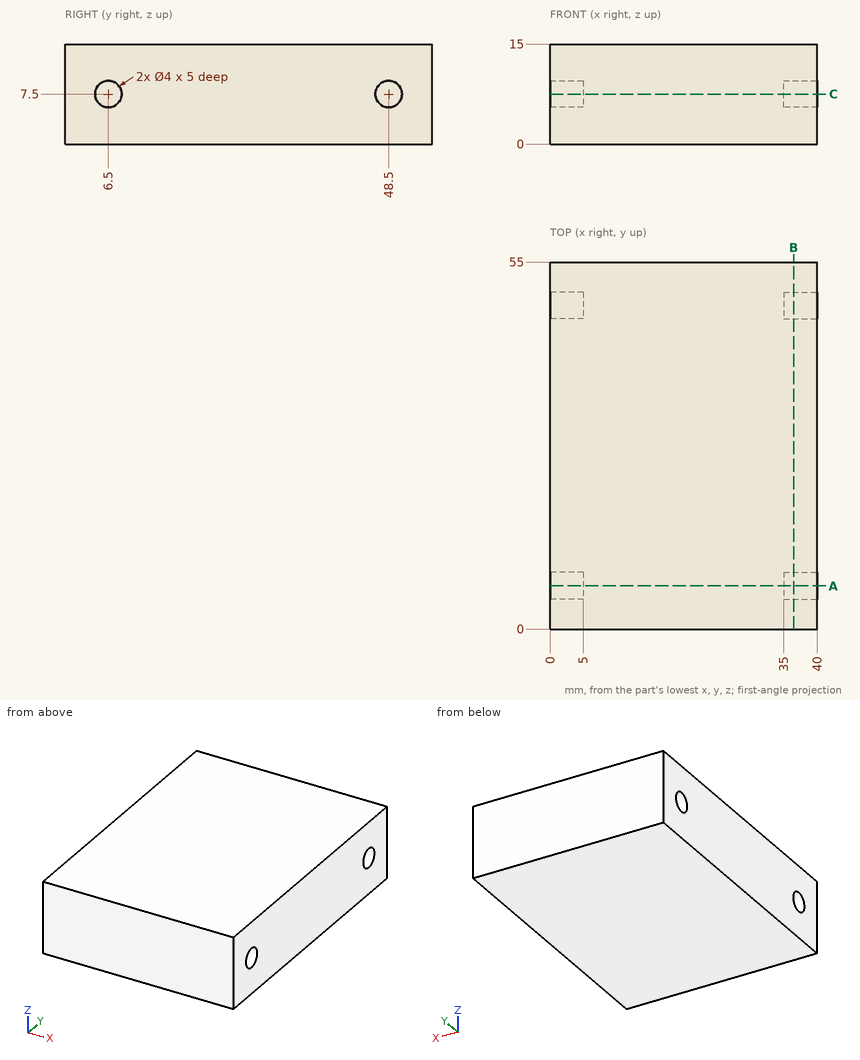
Could you check a few things on this drawing? It's one solid part, dimensions in mm from its lowest x, y, z. Coordinates: 2 decimals unless noted, no trailing zeros. Write each loop counter-clockwise with the first axis right and the second up, starting at its lowest first coordinate (ties: lowest second). Pieces come first, ordered by that corner, then holes. Notation, with made-up numbers: (65.5, -24.75) - (89.5, -24.75) arc R16 cw to (89.5, -19.75) - close; hole circle Ø4 at (11.5, 70.25). An arc over 180 degrees is marked (long way). Put each result on its own line as item: value. Start each with the question number.
Q1. I'm going to push flat-ended pins straight in: P1, Ø2.5, axis at y = 6.5, z = 7.5, coming from the +X side; P2, Ø1.2, axis at y = 49, z = 7, coming from the -X side. Where does each tip first touch, or does it pass through?
Q2. I want a section at C-C on z = 7.5. Write out the boundary of the cut face in (x, y).
Q3. Please list where these lines run through material, in increasing order: L1, parallel to Y at x = 37.45, z = 7.5; L2, parallel to Z at x = 36, y = 48; L3, parallel to Z at x = 2, y = 50.
Q4. I want a section at A-A on y = 6.5. Write out the boundary of the cut face in (x, z), plus the area to 3 significant figures.
Q5. I want a section at B-B on x = 36.5. Write out the boundary of the cut face in (y, z), plus the area to 3 significant figures.
Checks:
1. P1: x = 35
1. P2: x = 5
2. outline: (0, 0) - (40, 0) - (40, 4.5) - (35, 4.5) - (35, 8.5) - (40, 8.5) - (40, 46.5) - (35, 46.5) - (35, 50.5) - (40, 50.5) - (40, 55) - (0, 55) - (0, 50.5) - (5, 50.5) - (5, 46.5) - (0, 46.5) - (0, 8.5) - (5, 8.5) - (5, 4.5) - (0, 4.5) - close
3. L1: 0 to 4.5, 8.5 to 46.5, 50.5 to 55
3. L2: 0 to 5.56, 9.44 to 15
3. L3: 0 to 6.18, 8.82 to 15
4. outline: (0, 0) - (40, 0) - (40, 5.5) - (35, 5.5) - (35, 9.5) - (40, 9.5) - (40, 15) - (0, 15) - (0, 9.5) - (5, 9.5) - (5, 5.5) - (0, 5.5) - close
4. area: 560 mm²
5. outline: (0, 0) - (55, 0) - (55, 15) - (0, 15) - close; hole circle Ø4 at (6.5, 7.5); hole circle Ø4 at (48.5, 7.5)
5. area: 800 mm²
